from build123d import *

# Parameters (mm, degrees)
CYLINDER974_R             = 4.6
CYLINDER974_DEPTH         = 3.5
BOX564_W                  = 4.2
BOX564_H                  = 10
BOX564_DEPTH              = 5
BOX562_W                  = 10
BOX562_H                  = 4.2
BOX562_DEPTH              = 5
BOX563_W                  = 4.2
BOX563_H                  = 10
BOX563_DEPTH              = 5
BOX561_W                  = 10
BOX561_H                  = 4.2
BOX561_DEPTH              = 5
CYLINDER073_R             = 2.1
CYLINDER073_DEPTH         = 15
CYLINDER074_R             = 2.1
CYLINDER074_DEPTH         = 15
CYLINDER075_R             = 2.1
CYLINDER075_DEPTH         = 15
CYLINDER076_R             = 2.1
CYLINDER076_DEPTH         = 15
FUSION038_PLACEMENT_ANGLE = 90
CYLINDER961_R             = 1.6
CYLINDER961_DEPTH         = 15
CYLINDER962_R             = 1.6
CYLINDER962_DEPTH         = 15
CYLINDER963_R             = 1.6
CYLINDER963_DEPTH         = 15
CYLINDER959_R             = 1.6
CYLINDER959_DEPTH         = 15
CYLINDER960_R             = 1.6
CYLINDER960_DEPTH         = 15
BOX560_W                  = 26
BOX560_H                  = 22
BOX560_DEPTH              = 5


with BuildPart() as cylinder974:
    # Cylinder974 → Cylinder974 (new body)
    with BuildSketch(Plane.XY.offset(-3.5)):
        Circle(CYLINDER974_R)
    extrude(amount=CYLINDER974_DEPTH)


with BuildPart() as cube755:
    # Box564 → Box564 (new body)
    with BuildSketch(Plane(origin=(-2.1, -17, -2), x_dir=(1, 0, 0), z_dir=(0, 0, 1))):
        with Locations((2.1, 5)):
            Rectangle(BOX564_W, BOX564_H)
    extrude(amount=BOX564_DEPTH)


with BuildPart() as cube753:
    # Box562 → Box562 (new body)
    with BuildSketch(Plane(origin=(-17, -2.1, -2), x_dir=(1, 0, 0), z_dir=(0, 0, 1))):
        with Locations((5, 2.1)):
            Rectangle(BOX562_W, BOX562_H)
    extrude(amount=BOX562_DEPTH)


with BuildPart() as cube754:
    # Box563 → Box563 (new body)
    with BuildSketch(Plane(origin=(-2.1, 7, -2), x_dir=(1, 0, 0), z_dir=(0, 0, 1))):
        with Locations((2.1, 5)):
            Rectangle(BOX563_W, BOX563_H)
    extrude(amount=BOX563_DEPTH)


with BuildPart() as fusion107:
    # Box561 → Box561 (new body)
    with BuildSketch(Plane(origin=(7, -2.1, -2), x_dir=(1, 0, 0), z_dir=(0, 0, 1))):
        with Locations((5, 2.1)):
            Rectangle(BOX561_W, BOX561_H)
    extrude(amount=BOX561_DEPTH)

    # Fusion107: union Cube755, Cube753, Cube754
    add(cube755.part)
    add(cube753.part)
    add(cube754.part)


with BuildPart() as cylinder073:
    # Cylinder073 → Cylinder073 (new body)
    with BuildSketch(Plane(origin=(7, 0, 0), x_dir=(1, 0, 0), z_dir=(0, 0, 1))):
        Circle(CYLINDER073_R)
    extrude(amount=CYLINDER073_DEPTH)


with BuildPart() as fusion037:
    # Cylinder074 → Cylinder074 (new body)
    with BuildSketch(Plane(origin=(-7, 0, 0), x_dir=(1, 0, 0), z_dir=(0, 0, 1))):
        Circle(CYLINDER074_R)
    extrude(amount=CYLINDER074_DEPTH)

    # Fusion037: union Cylinder073
    add(cylinder073.part)


with BuildPart() as cylinder075:
    # Cylinder075 → Cylinder075 (new body)
    with BuildSketch(Plane(origin=(7, 0, 0), x_dir=(1, 0, 0), z_dir=(0, 0, 1))):
        Circle(CYLINDER075_R)
    extrude(amount=CYLINDER075_DEPTH)


with BuildPart() as fusion039:
    # Cylinder076 → Cylinder076 (new body)
    with BuildSketch(Plane(origin=(-7, 0, 0), x_dir=(1, 0, 0), z_dir=(0, 0, 1))):
        Circle(CYLINDER076_R)
    extrude(amount=CYLINDER076_DEPTH)

    # Fusion038: union Cylinder075
    add(cylinder075.part)


with BuildPart() as fusion039_1:
    # Fusion038 placement: moved
    add(fusion039.part.rotate(Axis((0, 0, 0), (0, 0, 1)), FUSION038_PLACEMENT_ANGLE))

    # Fusion039: union Fusion037
    add(fusion037.part)


with BuildPart() as fusion039_2:
    # Fusion039 placement: moved
    add(fusion039_1.part.moved(Location((0, 0, -3))))


with BuildPart() as cylinder961:
    # Cylinder961 → Cylinder961 (new body)
    with BuildSketch(Plane(origin=(-10, -8, -2), x_dir=(1, 0, 0), z_dir=(0, 0, 1))):
        Circle(CYLINDER961_R)
    extrude(amount=CYLINDER961_DEPTH)


with BuildPart() as cylinder962:
    # Cylinder962 → Cylinder962 (new body)
    with BuildSketch(Plane(origin=(10, 8, -2), x_dir=(1, 0, 0), z_dir=(0, 0, 1))):
        Circle(CYLINDER962_R)
    extrude(amount=CYLINDER962_DEPTH)


with BuildPart() as cylinder963:
    # Cylinder963 → Cylinder963 (new body)
    with BuildSketch(Plane(origin=(10, -8, -2), x_dir=(1, 0, 0), z_dir=(0, 0, 1))):
        Circle(CYLINDER963_R)
    extrude(amount=CYLINDER963_DEPTH)


with BuildPart() as cylinder959:
    # Cylinder959 → Cylinder959 (new body)
    with BuildSketch(Plane.XY.offset(-2)):
        Circle(CYLINDER959_R)
    extrude(amount=CYLINDER959_DEPTH)


with BuildPart() as fusion105:
    # Cylinder960 → Cylinder960 (new body)
    with BuildSketch(Plane(origin=(-10, 8, -2), x_dir=(1, 0, 0), z_dir=(0, 0, 1))):
        Circle(CYLINDER960_R)
    extrude(amount=CYLINDER960_DEPTH)

    # Fusion105: union Cylinder961, Cylinder962, Cylinder963, Cylinder959
    add(cylinder961.part)
    add(cylinder962.part)
    add(cylinder963.part)
    add(cylinder959.part)


with BuildPart() as diff_lock_planetary_sup_holes:
    # Box560 → Box560 (new body)
    with BuildSketch(Plane(origin=(-13, -11, -2), x_dir=(1, 0, 0), z_dir=(0, 0, 1))):
        with Locations((13, 11)):
            Rectangle(BOX560_W, BOX560_H)
    extrude(amount=BOX560_DEPTH)

    # Cut014050: cut Fusion105
    add(fusion105.part, mode=Mode.SUBTRACT)

    # Cut014051: cut Fusion039
    add(fusion039_2.part, mode=Mode.SUBTRACT)

    # Cut014055: cut Fusion107
    add(fusion107.part, mode=Mode.SUBTRACT)


with BuildPart() as diff_lock_planetary_sup_holes_1:
    # Cut014055 placement: moved
    add(diff_lock_planetary_sup_holes.part.moved(Location((0, 0, -3))))

    # Cut014056: cut Cylinder974
    add(cylinder974.part, mode=Mode.SUBTRACT)


solid = diff_lock_planetary_sup_holes_1.part
Geometry: final body of the model. Coordinates: model frame, mm. A direction names the side the tool comes from. Coordinates: 2 decimals unless noted, no trailing zeros. Loops run counter-clockwise (first coordinate to the right, second up) from the corner with the lowest first, then second, coordinate; pieces in that order, holes last. Notation, with made-up numbers: (-30, 25.25) - (-10, 25.25) arc R36 ccw to (-10, 59.25) - close; hole circle Ø11 at (-1, 72). An arc over 180 degrees is marked (long way). One line per question, with ' | ' between items. Start each with the question number.
(1) Cut plane C-C on z = -3.95. Output: boundary loops of the cut face in (x, y), and give its area (3 significant figures).
(2) Reachability of faces 1 (the cylindrical face through (-3.65, -2.8, -1.77)), 2 (the flat face through (-10, -2.1, -3)), 3 (the flat face through (-2.1, -9, -3)), 4 (the flat face through (-2.1, 9, -3)) from +Z, -Z, +X, -X, +Y, -Y: full face, straight path, thin tool, end or side. Return the list, or none.
(3) First-contact query: pin 1 (5 mm diameter, centred on x = 0, y = 0, fed in from +Z). Flat tip, straight axial feed; report the tip coordinate or a pass-through.
(4) Cut plane A-A on x = -10. Output: boundary loops of the cut face in (y, z).
(5) Ray query, L1, parallel to X at y = 8, z = -2.9; L2, parallel to Y at x = -10, z = -3.6; L3, parallel to Y at x = 7.25, z = -1.7. Return the intervals inside material, ascending. Write a range as from..to.
(6) Cut plane D-D on x = -6.5. Output: boundary loops of the cut face in (y, z).
(7) Cut plane B-B on y = -8. Output: boundary loops of the cut face in (x, z).
Here are the results:
1) outline: (-13, -11) - (-2.1, -11) - (-2.1, -7) arc R2.1 cw to (2.1, -7) - (2.1, -11) - (13, -11) - (13, -2.1) - (7, -2.1) arc R2.1 cw to (7, 2.1) - (13, 2.1) - (13, 11) - (2.1, 11) - (2.1, 7) arc R2.1 cw to (-2.1, 7) - (-2.1, 11) - (-13, 11) - (-13, 2.1) - (-7, 2.1) arc R2.1 cw to (-7, -2.1) - (-13, -2.1) - close; hole circle Ø3.2 at (-10, -8); hole circle Ø3.2 at (-10, 8); hole circle Ø3.2 at (0, 0); hole circle Ø3.2 at (10, -8); hole circle Ø3.2 at (10, 8) | area: 420 mm²
2) face 1: +Z | face 2: +Z, -Z, -X | face 3: +Z, -Z, -Y | face 4: +Z, -Z, +Y
3) pin 1: z = -3.5
4) outline: (-11, -5) - (-9.6, -5) - (-9.6, 0) - (-11, 0) - close; (-6.4, -5) - (-2.1, -5) - (-2.1, 0) - (-6.4, 0) - close; (2.1, -5) - (6.4, -5) - (6.4, 0) - (2.1, 0) - close; (9.6, -5) - (11, -5) - (11, 0) - (9.6, 0) - close
5) L1: -13..-11.6, -8.4..-2.1, 2.1..8.4, 11.6..13 | L2: -11..-9.6, -6.4..-2.1, 2.1..6.4, 9.6..11 | L3: -11..-2.1, 2.1..11
6) outline: (-11, -5) - (-2.04, -5) - (-2.04, 0) - (-11, 0) - close; (2.04, -5) - (11, -5) - (11, 0) - (2.04, 0) - close
7) outline: (-13, -5) - (-11.6, -5) - (-11.6, 0) - (-13, 0) - close; (-8.4, -5) - (-2.1, -5) - (-2.1, 0) - (-8.4, 0) - close; (2.1, -5) - (8.4, -5) - (8.4, 0) - (2.1, 0) - close; (11.6, -5) - (13, -5) - (13, 0) - (11.6, 0) - close
